```python
from build123d import *

# Parameters (mm, degrees)
F0_R     = 18
F1_DEPTH = 15
F2_R     = 9
F2_R_2   = 3.25
F3_DEPTH = 4
F4_DEPTH = 25


with BuildPart() as f1:
    # F0 (on Top) → F1 (new body)
    with BuildSketch(Plane.XY):
        Circle(F0_R)
    extrude(amount=F1_DEPTH)

    # F2 (on face) → F3 (cut)
    with BuildSketch(Plane.XY.offset(15)):
        Circle(F2_R)
        Circle(F2_R_2, mode=Mode.SUBTRACT)
    extrude(amount=-F3_DEPTH, mode=Mode.SUBTRACT)

    # F2 (on face) → F4 (cut)
    with BuildSketch(Plane.XY.offset(15)):
        Circle(F2_R_2)
    extrude(amount=-F4_DEPTH, mode=Mode.SUBTRACT)


solid = f1.part
```
For this review, take the finished solid that the model builds, in its own axes (mm). A direction names the side the tool comes from. Round coordinates to 2 decimals unless told otherwise and drop trailing zeros. Write each loop counter-clockwise with the first axis right and the second up, starting at its lowest first coordinate (ties: lowest second). Pieces come first, ordered by that corner, then holes. Notation, with made-up numbers: (-15.5, 13) - (-4.5, 13) arc R3 ccw to (-4.5, 18) - close; hole circle Ø5 at (61.5, -0.5). An arc over 180 degrees is marked (long way). Answer as CSV lines item,"result". Start each with the question number.
(1) Add section C-C, the plane x = -5. State the section outline as (y, z) points, plus the area to 3 significant figures.
(2) For pin 1 (11 mm diameter, centred on x = 0, y = 0, fed in from +Z); pin 2 (1.5 mm diameter, centred on y = -13, z = 5, fed in from +X); pin 3 (6 mm diameter, centred on x = -1, z = 11.5, fed in from -Y), all flat-tipped, find the tip position at first contact; note any pin that passes through.
(3) Add section D-D, the plane z = 12.5. State the section outline as (x, y) points, plus the area to 3 significant figures.
(4) Mouldability with a two-part tool opening along Y and no side actions: class faces 3 (the flat face through (0, -4, 0)), 4 (the cylindrical face through (-2.343, 17.847, 7.395)), 5 (the cylindrical face through (-2.579, -1.978, 5.577)) as +Y half, -Y half, draft (parallel to the pull), parting line (faces both ways), or undercut.
(5) For line 1 (Y direction, x = 0, z = 12.45); line 2 (Y direction, x = 0, z = 2.75); line 3 (X direction, y = -1.5, z = 10.5), list the stretches that pass through material, from the lowest coordinate up.
(6) Machinability: for faces 1 (the flat face through (-8.3, 4.3, 15)), 2 (the flat face through (0, -4, 11)), which of the approach directions +Z, -Z, +X, -X, +Y, -Y give a long, thin tool a straight path to every point of the face, cutting with its end or side? Answer none if there is none.
(7) Add section A-A, the plane x = 0. State the section outline as (y, z) points.
From the geometry:
1,outline,"(-17.29, 0) - (17.29, 0) - (17.29, 15) - (7.48, 15) - (7.48, 11) - (-7.48, 11) - (-7.48, 15) - (-17.29, 15) - close"
1,area,"459 mm²"
2,pin 1,"stops at z = 11"
2,pin 2,"stops at x = 13.19"
2,pin 3,"stops at y = -18"
3,outline,"circle Ø36 at (0, 0); hole circle Ø18 at (0, 0)"
3,area,"763 mm²"
4,face 3,"draft"
4,face 4,"parting line"
4,face 5,"undercut"
5,line 1,"y = -18 to -9, 9 to 18"
5,line 2,"y = -18 to -3.25, 3.25 to 18"
5,line 3,"x = -17.94 to -2.88, 2.88 to 17.94"
6,face 1,"+Z, +X, -X, +Y, -Y"
6,face 2,"+Z"
7,outline,"(-18, 0) - (-3.25, 0) - (-3.25, 11) - (-9, 11) - (-9, 15) - (-18, 15) - close; (3.25, 0) - (18, 0) - (18, 15) - (9, 15) - (9, 11) - (3.25, 11) - close"
